```python
from build123d import *

# Parameters (mm, degrees)
SKETCH1_W           = 53
SKETCH1_H           = 53
BOSS_EXTRUDE1_DEPTH = 30
SKETCH6_W           = 51
SKETCH6_H           = 51
CUT_EXTRUDE1_DEPTH  = 10
SKETCH7_W           = 41
SKETCH7_H           = 41
CUT_EXTRUDE2_DEPTH  = 10
SKETCH14_R          = 1.5
CUT_EXTRUDE4_DEPTH  = 78.575769413
FILLET1_R           = 1


with BuildPart() as part:
    # Sketch1 → Boss-Extrude1 (new body)
    with BuildSketch(Plane(origin=(0, 0, 0), x_dir=(1, 0, 0), z_dir=(0, 1, 0))):
        with Locations((26.5, -26.5)):
            Rectangle(SKETCH1_W, SKETCH1_H)
    extrude(amount=BOSS_EXTRUDE1_DEPTH)

    # Sketch6 → Cut-Extrude1 (cut)
    with BuildSketch(Plane(origin=(0, 30, 0), x_dir=(1, 0, 0), z_dir=(0, 1, 0))):
        with Locations((26.5, -26.5)):
            Rectangle(SKETCH6_W, SKETCH6_H)
    extrude(amount=-CUT_EXTRUDE1_DEPTH, mode=Mode.SUBTRACT)

    # Sketch7 → Cut-Extrude2 (cut)
    with BuildSketch(Plane(origin=(0, 20, 0), x_dir=(1, 0, 0), z_dir=(0, 1, 0))):
        with Locations((26.5, -26.5)):
            Rectangle(SKETCH7_W, SKETCH7_H)
    extrude(amount=-CUT_EXTRUDE2_DEPTH, mode=Mode.SUBTRACT)

    # Sketch14 → Cut-Extrude4 (cut, through all)
    with BuildSketch(Plane(origin=(0, 10, 0), x_dir=(1, 0, 0), z_dir=(0, 1, 0))):
        with Locations(Location((11, -11, 0), (0, 0, 270))):
            Circle(SKETCH14_R)
        with Locations(Location((42, -11, 0), (0, 0, 270))):
            Circle(SKETCH14_R)
        with Locations(Location((42, -42, 0), (0, 0, 270))):
            Circle(SKETCH14_R)
        with Locations(Location((11, -42, 0), (0, 0, 270))):
            Circle(SKETCH14_R)
    extrude(amount=-CUT_EXTRUDE4_DEPTH, mode=Mode.SUBTRACT)

    # Fillet1
    fillet1_edges = [part.edges().sort_by_distance(p)[0] for p in [
        (6, 15, 6),
        (47, 15, 6),
        (47, 15, 47),
        (6, 15, 47),
        (26.5, 20, 6),
        (6, 20, 26.5),
        (26.5, 20, 47),
        (47, 20, 26.5),
        (0, 15, 0),
        (53, 15, 0),
        (53, 15, 53),
        (0, 15, 53),
    ]]
    fillet(fillet1_edges, radius=FILLET1_R)


solid = part.part
```
Part model, mm, in its own coordinate system. A direction names the side the tool comes from. Give positions to 0.01 mm unless a question says otherwise; leave off trailing zeros. Loops run counter-clockwise (first coordinate to the right, second up) from the corner with the lowest first, then second, coordinate; pieces in that order, holes last. Notation, with made-up numbers: M 57.5,82.25 L 103.5,82.25 A7 cw 103.5,91.25 Z; hole C -30.5,-1.75 d5. An arc over 180 degrees is marked long. Return JSON: item names as keys, results as strings.
1) Saw through at B-B, the plane z = 42. List the corners of the cut face in (x, y), then the cut area to 3 significant figures.
Calculated:
{"outline": "M 0,0 L 9.5,0 L 9.5,10 L 6,10 L 6,19 A1 ccw 5,20 L 1,20 L 1,30 L 0,30 Z; M 12.5,0 L 40.5,0 L 40.5,10 L 12.5,10 Z; M 43.5,0 L 53,0 L 53,30 L 52,30 L 52,20 L 48,20 A1 ccw 47,19 L 47,10 L 43.5,10 Z", "area": "610 mm2"}
2) Saw through at A-A, the plane x = 11. List the corners of the cut face in (y, z), then the cut area to 3 significant figures.
Calculated:
{"outline": "M 0,0 L 30,0 L 30,1 L 20,1 L 20,5 A1 ccw 19,6 L 10,6 L 10,9.5 L 0,9.5 Z; M 0,12.5 L 10,12.5 L 10,40.5 L 0,40.5 Z; M 0,43.5 L 10,43.5 L 10,47 L 19,47 A1 ccw 20,48 L 20,52 L 30,52 L 30,53 L 0,53 Z", "area": "610 mm2"}
3) Saw through at C-C, the plane z = 49. List the corners of the cut face in (x, y), then the cut area to 3 significant figures.
Calculated:
{"outline": "M 0,0 L 53,0 L 53,30 L 52,30 L 52,20 L 1,20 L 1,30 L 0,30 Z", "area": "1,080 mm2"}
4) Flat gauge pin, fed straight in: pin 1 Ø5 at (x, z) = (41, 11) entering from +Y. Where does the tip first touch, or does it go through?
Calculated:
{"pin 1": "stops at y = 10"}
5) 3-axis set-ups, long thin cutter, end or side, ignore diameter. For faces 1 (the face through (26, 10, 26)), 2 (the face through (40.536, 5.07, 10.675)): which of +Z, -Z, +X, -X, +Y, -Y reach the whole face in a straight line?
Calculated:
{"face 1": "+Y", "face 2": "+Y, -Y"}
6) Saw through at D-D, the plane z = 20. List the corners of the cut face in (x, y).
Calculated:
{"outline": "M 0,0 L 53,0 L 53,30 L 52,30 L 52,20 L 48,20 A1 ccw 47,19 L 47,10 L 6,10 L 6,19 A1 ccw 5,20 L 1,20 L 1,30 L 0,30 Z"}
7) Drill centre lines: line 1 (X direction, y = 7.5, z = 42); line 2 (Z direction, x = 46, y = 21.75). Where is each one in solid material? Low to high.
Calculated:
{"line 1": "x = 0 to 9.5, 12.5 to 40.5, 43.5 to 53", "line 2": "z = 0 to 1, 52 to 53"}
8) Pull direction X, two halves, no side cores. Call faces 3 (the face through (53, 15, 27)), 4 (the face through (0, 15, 27)), 5 (the face through (26, 15, 53)), 6 (the face through (26, 25, 52)): released by +X, released by -X, zero draft, split by the parting line, or undercut.
Calculated:
{"face 3": "released by +X", "face 4": "released by -X", "face 5": "zero draft", "face 6": "undercut"}
